from build123d import *

# Parameters (mm, degrees)
SKETCH_1_W      = 85
SKETCH_1_H      = 13
SKETCH_1_R      = 2.55
SKETCH_1_W_2    = 7.8
SKETCH_1_H_2    = 4.8
SKETCH_1_W_3    = 7.6
SKETCH_1_H_3    = 3
SKETCH_1_W_4    = 11.2
EXTRUDE_2_DEPTH = 2


with BuildPart() as part:
    # 草图1 → 凸台-拉伸2 (new body)
    with BuildSketch(Plane(origin=(0, 0, 0), x_dir=(1, 0, 0), z_dir=(0, 1, 0))):
        with Locations((32.448630137, -1.668848032)):
            Rectangle(SKETCH_1_W, SKETCH_1_H)
        with Locations(Location((39.591348171, -1.868848032, 0), (0, 0, 270))):
            Circle(SKETCH_1_R, mode=Mode.SUBTRACT)
        with Locations((64.891348171, -1.968848032)):
            Rectangle(SKETCH_1_W_2, SKETCH_1_H_2, mode=Mode.SUBTRACT)
        with Locations((52.191348171, -1.668848032)):
            Rectangle(SKETCH_1_W_3, SKETCH_1_H_3, mode=Mode.SUBTRACT)
        with Locations((24.191348171, -0.668848032)):
            Rectangle(SKETCH_1_W_4, SKETCH_1_H_3, mode=Mode.SUBTRACT)
        with Locations((7.591348171, -0.668848032)):
            Rectangle(SKETCH_1_W_4, SKETCH_1_H_3, mode=Mode.SUBTRACT)
    extrude(amount=EXTRUDE_2_DEPTH)


solid = part.part
CAD build for the part. Positions are in the model's coordinates, mm. A direction names the side the tool comes from. Round coordinates to 2 decimals unless told otherwise and drop trailing zeros. Order: outer loops, then holes, each group sorted by start corner. A loop starts at its lowest first (then second) coordinate and runs counter-clockwise, first axis right, second up. Notation, with made-up numbers: (56.5, 28) -> (88.5, 28) arc R24 ccw to (88.5, 51) -> close; hole circle Ø10 at (24, 83.25). An arc over 180 degrees is marked (long way). Write each question's results on one line, items separated by ' | '.
1. Pull direction Z, two halves, no side cores. Call faces 3 (the face through (55.991, 1, 2)), 4 (the face through (32, 1, -4.831)), 5 (the face through (32, 0, 2)): pulls with the +Z half, pulls with the -Z half, needs draft (parallel to the pull), parting line crosses it, or undercut.
Findings below:
face 3: undercut | face 4: pulls with the -Z half | face 5: needs draft
2. Wall check: line 1 along X through (y, z) = (1.1, 2.75); line 2 along X through (y, z) = (0.9, 0); line 3 along Z through (x, y) = (2.5, 1.5). Give the ranges that are in metal, low to high. Write a range as [from, to].
Findings below:
line 1: x = [-10.05, 37.2], [41.98, 48.39], [55.99, 60.99], [68.79, 74.95] | line 2: x = [-10.05, 1.99], [13.19, 18.59], [29.79, 37.86], [41.33, 60.99], [68.79, 74.95] | line 3: z = [-4.83, -0.83], [2.17, 8.17]
3. Cut at C-C (x = 62). Give the cut face in (y, z).
Findings below:
outline: (0, -4.83) -> (2, -4.83) -> (2, -0.43) -> (0, -0.43) -> close; (0, 4.37) -> (2, 4.37) -> (2, 8.17) -> (0, 8.17) -> close
4. Cut at B-B (y = 1.45). Give the cut face in (x, z).
Findings below:
outline: (-10.05, -4.83) -> (74.95, -4.83) -> (74.95, 8.17) -> (-10.05, 8.17) -> close; hole (1.99, -0.83) -> (13.19, -0.83) -> (13.19, 2.17) -> (1.99, 2.17) -> close; hole (18.59, -0.83) -> (29.79, -0.83) -> (29.79, 2.17) -> (18.59, 2.17) -> close; hole circle Ø5.1 at (39.59, 1.87); hole (48.39, 0.17) -> (55.99, 0.17) -> (55.99, 3.17) -> (48.39, 3.17) -> close; hole (60.99, -0.43) -> (68.79, -0.43) -> (68.79, 4.37) -> (60.99, 4.37) -> close
5. Cut at A-A (x = 22). Give the cut face in (y, z), plus the area to 3 significant figures.
Findings below:
outline: (0, -4.83) -> (2, -4.83) -> (2, -0.83) -> (0, -0.83) -> close; (0, 2.17) -> (2, 2.17) -> (2, 8.17) -> (0, 8.17) -> close | area: 20.0 mm²
6. 3-axis set-ups, long thin cutter, end or side, ignore diameter. For faces 1 (the face through (65, 1, -0.431)), 2 (the face through (32, 2, 2)): which of +Z, -Z, +X, -X, +Y, -Y reach the whole face in a straight line?
Findings below:
face 1: +Y, -Y | face 2: +Z, -Z, +X, -X, +Y
